Verification items for the finished model (mm, model axes). Round coordinates to 2 decimals unless told otherwise and drop trailing zeros. Write each loop counter-clockwise with the first axis right and the second up, starting at its lowest first coordinate (ties: lowest second). Pieces come first, ordered by that corner, then holes. Notation, with made-up numbers: (-6.5, 38.25) - (8.5, 38.25) arc R23 cw to (8.5, 54.25) - close; hole circle Ø9 at (63, 70.5). An arc over 180 degrees is marked (long way). Answer as a JSON object with one key per item and string values. Group by question number.
1) Section check A-A (z = 1.1). State how many separate pieces and enclosed holes the cut face has, then the cut area to 3 significant figures.
2) Thickness scan on line 1 (Y direction, x = -40, z = 2.1); line 2 (Y direction, x = 0, z = 2.3); line 3 (X direction, y = 1, z = 2). Record the ranges inside material, lowest first.
3) Section check B-B (y = -47.5). Enter the section's corners in (x, z), then the cut area to 3 significant figures.
4) Go/stop test with flat-tipped pins: pin 1 Ø2.5 at (x, y) = (-28.79, -12.1) entering from +Z; pin 2 Ø1 at (x, z) = (-12, 2.5) entering from +Y. Record where each tip stops, or that it passes through.
```python
from build123d import *

# Parameters (mm, degrees)
SKETCH2_R           = 1.5
BOSS_EXTRUDE2_DEPTH = 3


with BuildPart() as part:
    # Sketch2 → Boss-Extrude2 (new body)
    with BuildSketch(Plane.XY):
        with BuildLine():
            Line((-50, -13.815728753), (-50, 13.815728753))
            ThreePointArc((-50, 13.815728753), (-48.47759065, 21.4693974), (-44.142135624, 27.957864376))
            Line((-44.142135624, 27.957864376), (-34.644660941, 37.455339059))
            ThreePointArc((-34.644660941, 37.455339059), (-30.309205914, 43.943806036), (-28.786796564, 51.597474683))
            Line((-28.786796564, 51.597474683), (-28.786796564, 70))
            ThreePointArc((-28.786796564, 70), (-22.928932188, 84.142135624), (-8.786796564, 90))
            Line((-8.786796564, 90), (8.786796564, 90))
            ThreePointArc((8.786796564, 90), (22.928932188, 84.142135624), (28.786796564, 70))
            Line((28.786796564, 70), (28.786796564, 51.597474683))
            ThreePointArc((28.786796564, 51.597474683), (30.309205914, 43.943806036), (34.644660941, 37.455339059))
            Line((34.644660941, 37.455339059), (44.142135624, 27.957864376))
            ThreePointArc((44.142135624, 27.957864376), (48.47759065, 21.4693974), (50, 13.815728753))
            Line((50, 13.815728753), (50, -13.815728753))
            ThreePointArc((50, -13.815728753), (48.47759065, -21.4693974), (44.142135624, -27.957864376))
            Line((44.142135624, -27.957864376), (34.644660941, -37.455339059))
            ThreePointArc((34.644660941, -37.455339059), (30.309205914, -43.943806036), (28.786796564, -51.597474683))
            Line((28.786796564, -51.597474683), (28.786796564, -70))
            ThreePointArc((28.786796564, -70), (22.928932188, -84.142135624), (8.786796564, -90))
            Line((8.786796564, -90), (-8.786796564, -90))
            ThreePointArc((-8.786796564, -90), (-22.928932188, -84.142135624), (-28.786796564, -70))
            Line((-28.786796564, -70), (-28.786796564, -51.597474683))
            ThreePointArc((-28.786796564, -51.597474683), (-30.309205914, -43.943806036), (-34.644660941, -37.455339059))
            Line((-34.644660941, -37.455339059), (-44.142135624, -27.957864376))
            ThreePointArc((-44.142135624, -27.957864376), (-48.47759065, -21.4693974), (-50, -13.815728753))
        make_face()
        with Locations((0, 85)):
            Circle(SKETCH2_R, mode=Mode.SUBTRACT)
        with Locations((-23.786796564, 66.656601718)):
            Circle(SKETCH2_R, mode=Mode.SUBTRACT)
        with Locations((-28.786796564, 32.1)):
            Circle(SKETCH2_R, mode=Mode.SUBTRACT)
        with Locations((-38.786796564, 22.1)):
            Circle(SKETCH2_R, mode=Mode.SUBTRACT)
        with Locations((-28.786796564, 12.1)):
            Circle(SKETCH2_R, mode=Mode.SUBTRACT)
        with Locations((-18.786796564, 22.1)):
            Circle(SKETCH2_R, mode=Mode.SUBTRACT)
        with Locations((-45, 0)):
            Circle(SKETCH2_R, mode=Mode.SUBTRACT)
        with Locations(Location((45, 0, 0), (0, 0, 180))):
            Circle(SKETCH2_R, mode=Mode.SUBTRACT)
        with Locations(Location((18.786796564, 22.1, 0), (0, 0, 180))):
            Circle(SKETCH2_R, mode=Mode.SUBTRACT)
        with Locations(Location((28.786796564, 12.1, 0), (0, 0, 180))):
            Circle(SKETCH2_R, mode=Mode.SUBTRACT)
        with Locations(Location((38.786796564, 22.1, 0), (0, 0, 180))):
            Circle(SKETCH2_R, mode=Mode.SUBTRACT)
        with Locations(Location((28.786796564, 32.1, 0), (0, 0, 180))):
            Circle(SKETCH2_R, mode=Mode.SUBTRACT)
        with Locations(Location((23.786796564, 66.656601718, 0), (0, 0, 180))):
            Circle(SKETCH2_R, mode=Mode.SUBTRACT)
        with Locations((28.786796564, -32.1)):
            Circle(SKETCH2_R, mode=Mode.SUBTRACT)
        with Locations((38.786796564, -22.1)):
            Circle(SKETCH2_R, mode=Mode.SUBTRACT)
        with Locations((28.786796564, -12.1)):
            Circle(SKETCH2_R, mode=Mode.SUBTRACT)
        with Locations((18.786796564, -22.1)):
            Circle(SKETCH2_R, mode=Mode.SUBTRACT)
        with Locations(Location((-18.786796564, -22.1, 0), (0, 0, 180))):
            Circle(SKETCH2_R, mode=Mode.SUBTRACT)
        with Locations(Location((-28.786796564, -12.1, 0), (0, 0, 180))):
            Circle(SKETCH2_R, mode=Mode.SUBTRACT)
        with Locations(Location((-38.786796564, -22.1, 0), (0, 0, 180))):
            Circle(SKETCH2_R, mode=Mode.SUBTRACT)
        with Locations(Location((-28.786796564, -32.1, 0), (0, 0, 180))):
            Circle(SKETCH2_R, mode=Mode.SUBTRACT)
        with Locations((23.786796564, -66.656601718)):
            Circle(SKETCH2_R, mode=Mode.SUBTRACT)
        with Locations(Location((-23.786796564, -66.656601718, 0), (0, 0, 180))):
            Circle(SKETCH2_R, mode=Mode.SUBTRACT)
        with Locations(Location((0, -85, 0), (0, 0, 180))):
            Circle(SKETCH2_R, mode=Mode.SUBTRACT)
    extrude(amount=BOSS_EXTRUDE2_DEPTH)


solid = part.part
```
Returned:
{
 "1": {"separate pieces": "1", "enclosed holes": "24", "area": "12,600 mm2"},
 "2": {"line 1": "-32.1 to -22.98, -21.22 to 21.22, 22.98 to 32.1", "line 2": "-90 to -86.5, -83.5 to 83.5, 86.5 to 90", "line 3": "-50 to -46.12, -43.88 to 43.88, 46.12 to 50"},
 "3": {"outline": "(-29.21, 0) - (29.21, 0) - (29.21, 3) - (-29.21, 3) - close", "area": "175 mm2"},
 "4": {"pin 1": "through", "pin 2": "y = 89.82"}
}
